Design review of the part built by this model. Coordinates are the model's own, in mm. Face numbers are marked on the shaded views. A direction names the side the tool comes from. Give positions to 0.01 mm unless a question says otherwise; leave off trailing zeros. Order: outer loops, then holes, each group sorted by start corner. A loop starts at its lowest first (then second) coordinate and runs counter-clockwise, first axis right, second up. Notation, with made-up numbers: (24, 23) -> (64, 23) arc R13 ccw to (64, 48) -> close; hole circle Ø11 at (62, -16). An arc over 180 degrees is marked (long way). Return JSON: item names as keys, results as strings.
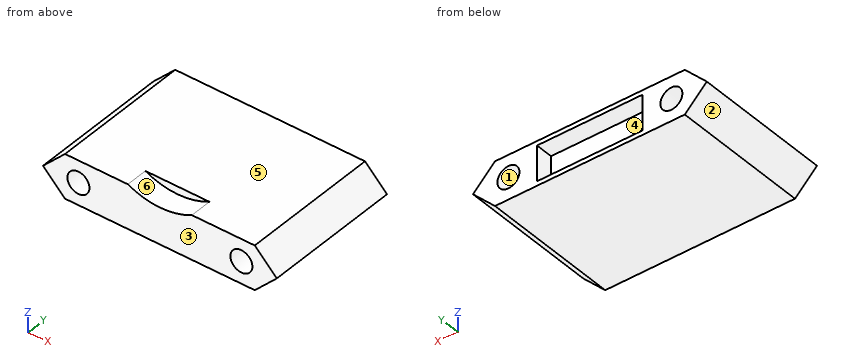
```python
from build123d import *

# Parameters (mm, degrees)
SKETCH1_R           = 3.175
BOSS_EXTRUDE1_DEPTH = 40
SKETCH2_W           = 30.48
SKETCH2_H           = 10.16
CUT_EXTRUDE1_DEPTH  = 5.08
SKETCH3_R           = 20.32
CUT_EXTRUDE2_DEPTH  = 6.35


with BuildPart() as part:
    # Sketch1 → Boss-Extrude1 (new body)
    with BuildSketch(Plane(origin=(0, 0, 0), x_dir=(1, 0, 0), z_dir=(0, 1, 0))):
        Polygon((-27.358849143, 6.35), (-33.708849143, 0), (-27.358849143, -6.35), (27.358849143, -6.35), (33.708849143, 0), (27.358849143, 6.35), align=None)
        with Locations((-23.495, 0)):
            Circle(SKETCH1_R, mode=Mode.SUBTRACT)
        with Locations((23.495, 0)):
            Circle(SKETCH1_R, mode=Mode.SUBTRACT)
    extrude(amount=BOSS_EXTRUDE1_DEPTH)

    # Sketch2 → Cut-Extrude1 (cut)
    with BuildSketch(Plane(origin=(0, 40, 0), x_dir=(1, 0, 0), z_dir=(0, 1, 0))):
        Rectangle(SKETCH2_W, SKETCH2_H)
    extrude(amount=-CUT_EXTRUDE1_DEPTH, mode=Mode.SUBTRACT)

    # Sketch3 → Cut-Extrude2 (cut)
    with BuildSketch(Plane(origin=(0, 0, 0), x_dir=(-1, 0, 0), z_dir=(0, -1, 0))):
        with Locations((0, -24.45005636)):
            Circle(SKETCH3_R)
    extrude(amount=-CUT_EXTRUDE2_DEPTH, mode=Mode.SUBTRACT)


solid = part.part
```
Item 1: Machinability: for the marked faces 4, 5 and 6, which of the approach directions +Z, -Z, +X, -X, +Y, -Y give a long, thin tool a straight path to every point of the face, cutting with its end or side? Answer none if there is none.
Result set:
{"face 4": "+Y", "face 5": "+Z, +X, -X, +Y, -Y", "face 6": "+Z, -Y"}
Item 2: Add section B-B (z = -1.25). Give the boundary of the cut face in (x, y).
Result set:
{"outline": "(-32.46, 0) -> (-26.41, 0) -> (-26.41, 40) -> (-32.46, 40) -> close; (-20.58, 0) -> (20.58, 0) -> (20.58, 40) -> (15.24, 40) -> (15.24, 34.92) -> (-15.24, 34.92) -> (-15.24, 40) -> (-20.58, 40) -> close; (26.41, 0) -> (32.46, 0) -> (32.46, 40) -> (26.41, 40) -> close"}
Item 3: Add section A-A (y = 31). Give the boundary of the cut face in (x, z) (3 decimals).
Result set:
{"outline": "(-33.709, 0) -> (-27.359, -6.35) -> (27.359, -6.35) -> (33.709, 0) -> (27.359, 6.35) -> (-27.359, 6.35) -> close; hole circle Ø6.35 at (-23.495, 0); hole circle Ø6.35 at (23.495, 0)"}
Item 4: Mouldability with a two-part tool opening along Z and no side actions: class the marked faces 1, 2 and 3 as released by +Z, released by -Z, zero draft, split by the parting line, or undercut.
Result set:
{"face 1": "undercut", "face 2": "released by -Z", "face 3": "zero draft"}
Item 5: Wall thickness on L1, parallel to X at y = 28.5, z = 2; L2, parallel to Z at x = 23.5, y = 32 (3 decimals); L3, parallel to X at y = 37, z = 1.5: over which ranges is each line inside the solid? List them lowest first. Write a range as [from, to].
Result set:
{"L1": "x = [-31.71, -25.96], [-21.03, 21.03], [25.96, 31.71]", "L2": "z = [-6.35, -3.175], [3.175, 6.35]", "L3": "x = [-32.21, -26.29], [-20.7, -15.24], [15.24, 20.7], [26.29, 32.21]"}
Item 6: Add section D-D (x = -10). Give the boundary of the cut face in (y, z), plus the area to 3 significant figures.
Result set:
{"outline": "(0, -6.35) -> (40, -6.35) -> (40, -5.08) -> (34.92, -5.08) -> (34.92, 5.08) -> (40, 5.08) -> (40, 6.35) -> (0, 6.35) -> close", "area": "456 mm^2"}
Item 7: For pin 1 (5 mm diameter, centred on x = 5, z = -2, fed in from +Y); pin 2 (2.5 mm diameter, centred on x = 0, z = 5, fed in from -Y); pin 3 (5 mm diameter, centred on x = 23.495, z = 0, fed in from +Y); pin 4 (4 mm diameter, centred on y = 37.5, z = 2.5, fed in from +X), all flat-tipped, find the tip position at first contact; note any pin that passes through.
Result set:
{"pin 1": "stops at y = 34.92", "pin 2": "stops at y = 0", "pin 3": "passes through", "pin 4": "stops at x = 33.21"}
Item 8: Add section C-C (x = 25.5). Give the boundary of the cut face in (y, z).
Result set:
{"outline": "(0, -6.35) -> (40, -6.35) -> (40, -2.46) -> (0, -2.46) -> close; (0, 2.46) -> (40, 2.46) -> (40, 6.35) -> (0, 6.35) -> close"}
